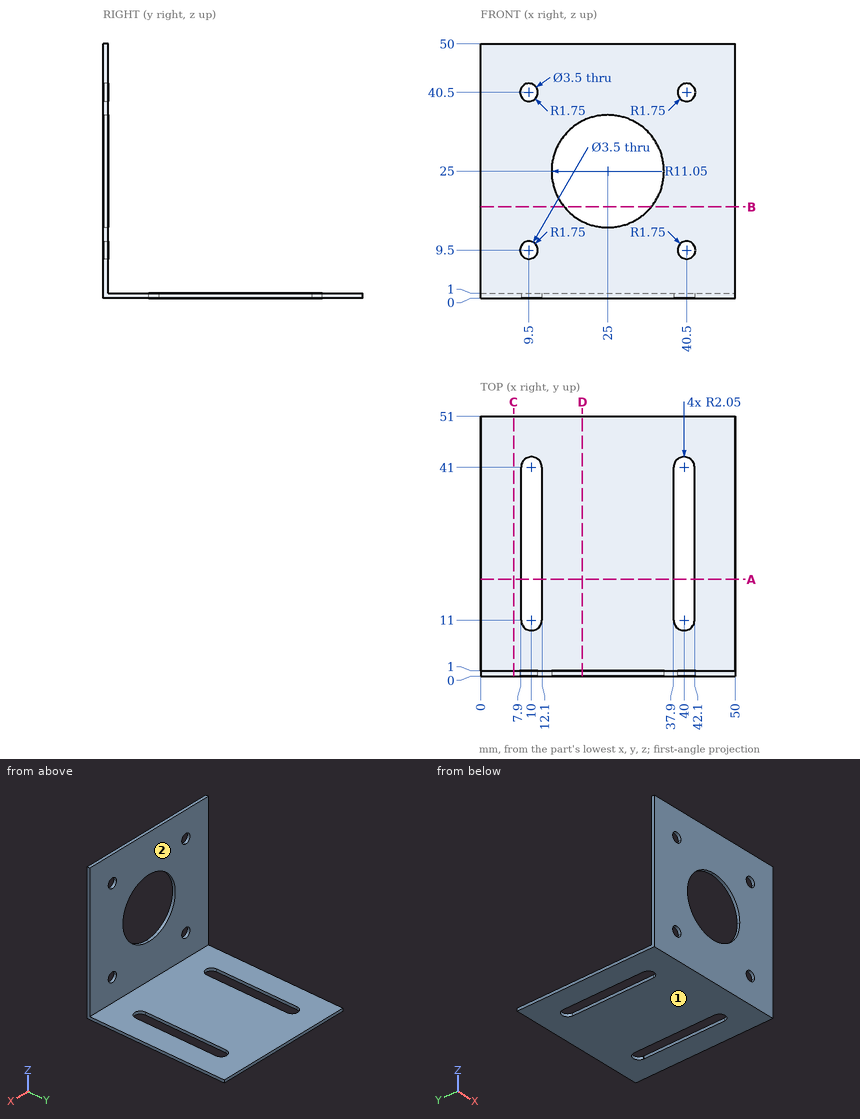
Input: dimensioned drawing with shaded views. Units: mm. Origin: part minimum x, y, z. A direction names the side the tool comes from. Give positions to 0.01 mm unless a question says otherwise; leave off trailing zeros. Write each loop counter-clockwise with the first axis right and the second up, starting at its lowest first coordinate (ties: lowest second). Pieces come first, ordered by that corner, then holes. Notation, with made-up numbers: (32, 4) -> (63, 4) arc R22 ccw to (63, 17) -> close; hole circle Ø6 at (-9, 58). An arc over 180 degrees is marked (long way). Answer as a JSON object with one key per item and string values.
1. Cut plane B-B on z = 18. Output: boundary loops of the cut face in (x, y).
Ans:
{"outline": "(0, 0) -> (16.45, 0) -> (16.45, 1) -> (0, 1) -> close; (33.55, 0) -> (50, 0) -> (50, 1) -> (33.55, 1) -> close"}
2. Contact query for flat-ended pins moving along their axis: pin 1 (2 mm diameter, centred on x = 9.5, z = 9.5, fed in from +Y); pin 2 (2 mm diameter, centred on x = 32, z = 16.5, fed in from -Y); pin 3 (4 mm diameter, centred on x = 44, y = 23, fed in from +Z). Output: stop coordinate, or through.
Ans:
{"pin 1": "passes through", "pin 2": "stops at y = 0", "pin 3": "stops at z = 1"}
3. Cut plane D-D on x = 20. Output: boundary loops of the cut face in (y, z).
Ans:
{"outline": "(0, 0) -> (51, 0) -> (51, 1) -> (1, 1) -> (1, 15.15) -> (0, 15.15) -> close; (0, 34.85) -> (1, 34.85) -> (1, 50) -> (0, 50) -> close"}
4. Cut plane C-C on x = 6.5. Output: boundary loops of the cut face in (y, z), and give its area (3 significant figures).
Ans:
{"outline": "(0, 0) -> (51, 0) -> (51, 1) -> (1, 1) -> (1, 50) -> (0, 50) -> close", "area": "100 mm^2"}
5. Cut plane A-A on y = 19. Output: boundary loops of the cut face in (x, z).
Ans:
{"outline": "(0, 0) -> (7.9, 0) -> (7.9, 1) -> (0, 1) -> close; (12.1, 0) -> (37.9, 0) -> (37.9, 1) -> (12.1, 1) -> close; (42.1, 0) -> (50, 0) -> (50, 1) -> (42.1, 1) -> close"}
6. Access query for the marked faces 1 and 2. Directions: +Z, -Z, +X, -X, +Y, -Y. A direction counts if a zero-diameter tool reaches every point of the face in a straight line with its end or side. Return the directions, or none.
Ans:
{"face 1": "-Z, +X, -X, +Y, -Y", "face 2": "+Z, +X, -X, +Y"}
7. Ray query, probe 1 along X at (y, z) = (0.75, 40.5); probe 2 along Y at (x, z) = (36, 37.5). Return the intervals inside material, ascending. Write a range as from..to.
Ans:
{"probe 1": "x = 0..7.75, 11.25..38.75, 42.25..50", "probe 2": "y = 0..1"}
